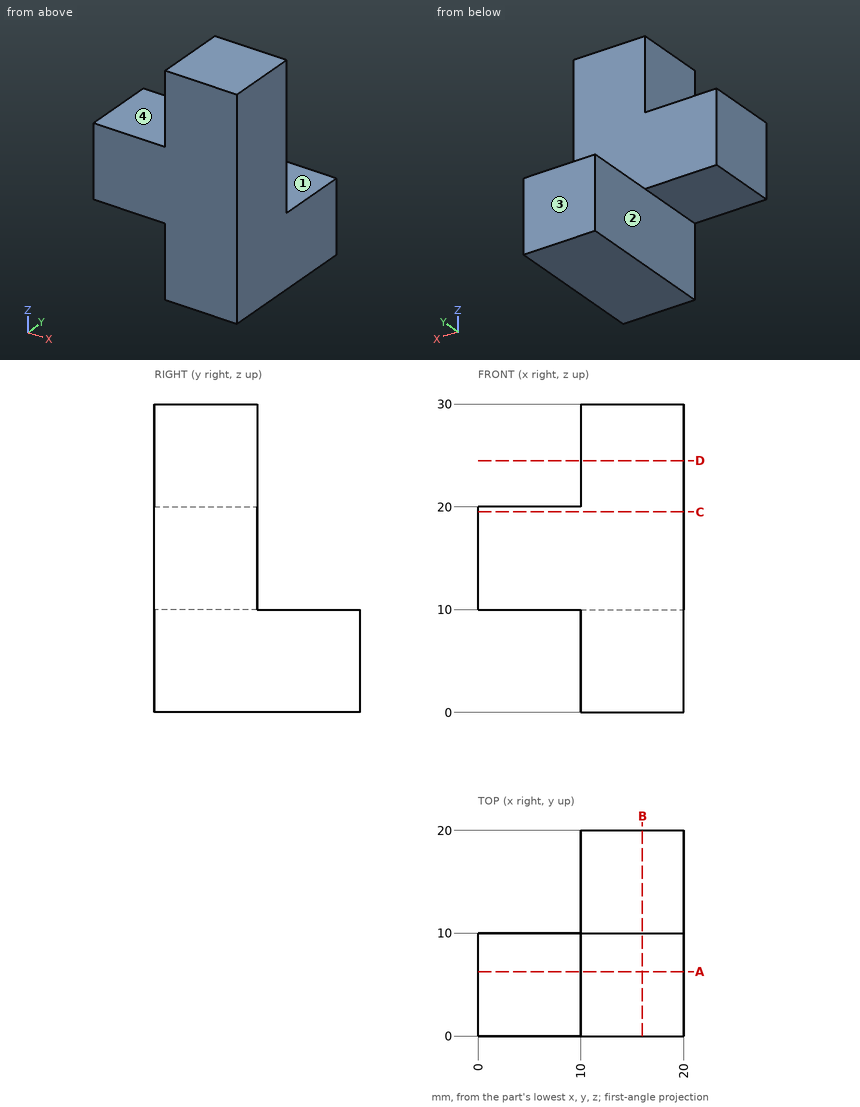
Could you check a few things on this drawing? It's one solid part, dimensions in mm from its lowest x, y, z. A direction names the side the tool comes from. Coordinates: 2 decimals unless noted, no trailing zeros. Order: outer loops, then holes, each group sorted by start corner. A loop starts at its lowest first (then second) coordinate and runs counter-clockwise, first axis right, second up. Notation, with made-up numbers: (87, -3.75) -> (120, -3.75) arc R28 ccw to (120, 24.25) -> close; hole circle Ø9 at (23.25, 0). An arc over 180 degrees is marked (long way). Answer in a Markdown table with one row per item.
(1) Will these pins go through, and if not, where does the flat tip stop? pin 1 Ø10 at (x, z) = (8, 24) entering from +Y; pin 2 Ø8 at (x, y) = (5, 5.5) entering from +Z; pin 3 Ø8 at (y, z) = (6, 25.5) entering from -X.
Answer key:
| item | result |
|---|---|
| pin 1 | y = 10 |
| pin 2 | z = 20 |
| pin 3 | x = 10 |
(2) On a 3-axis mill with a long thin cutter (end or side, diameter ignored), from which of +Z, -Z, +X, -X, +Y, -Y can I reach the whole of each face in a straight line? I mean the marked faces 1, 2, 3 and 4. Say none if no direction works.
Answer key:
| item | result |
|---|---|
| face 1 | +Z, +X, -X, +Y |
| face 2 | -Z, -X, +Y, -Y |
| face 3 | +Z, -Z, +X, -X, +Y |
| face 4 | +Z, -X, +Y, -Y |
(3) Please list where these lines run through material, in increasing order: probe 1 along Y at (x, z) = (10.75, 17); probe 2 along Z at (x, y) = (2.5, 3).
Answer key:
| item | result |
|---|---|
| probe 1 | 0 to 10 |
| probe 2 | 10 to 20 |
(4) I want a section at C-C on z = 19.5. List the corners of the cut face in (x, y) for me, then the cut area to 3 significant figures.
Answer key:
| item | result |
|---|---|
| outline | (0, 0) -> (20, 0) -> (20, 10) -> (0, 10) -> close |
| area | 200 mm^2 |
(5) I want a section at D-D on z = 24.5. List the corners of the cut face in (x, y) for me, then the cut area to 3 significant figures.
Answer key:
| item | result |
|---|---|
| outline | (10, 0) -> (20, 0) -> (20, 10) -> (10, 10) -> close |
| area | 100 mm^2 |
(6) I want a section at B-B on x = 16. List the corners of the cut face in (y, z) for me, then the cut area to 3 significant figures.
Answer key:
| item | result |
|---|---|
| outline | (0, 0) -> (20, 0) -> (20, 10) -> (10, 10) -> (10, 30) -> (0, 30) -> close |
| area | 400 mm^2 |
(7) I want a section at A-A on y = 6.25. List the corners of the cut face in (x, z) for me.
Answer key:
| item | result |
|---|---|
| outline | (0, 10) -> (10, 10) -> (10, 0) -> (20, 0) -> (20, 30) -> (10, 30) -> (10, 20) -> (0, 20) -> close |
